Check sheet for the drawn part. Datum: minimum x, y, z corner. Units: mm. A direction names the side the tool comes from. Coordinates: 2 decimals unless noted, no trailing zeros. Loops run counter-clockwise (first coordinate to the right, second up) from the corner with the lowest first, then second, coordinate; pieces in that order, holes last. Notation, with made-up numbers: (75, 50.25) -> (103, 50.25) arc R22 ccw to (103, 72.25) -> close; hole circle Ø1 at (20, 43). An arc over 180 degrees is marked (long way). Use CSV: the item, a comma, the result in double quotes. Start each with the question number.
1. Gauge pin test, flat ends, axial feed: pin 1 (2 mm diameter, centred on x = 54.5, z = 75, fed in from +Y) (3 decimals); pin 2 (18 mm diameter, centred on x = 89, y = 171, fed in from +Z); pin 3 (5 mm diameter, centred on y = 103.5, z = 72, fed in from +X). Record the tip position at first contact, or that the pin passes through.
2. Sectioned sample at B-B, the plane x = 81. Record the cut outline in (y, z).
3. Sectioned sample at D-D, the plane y = 166.5. Record the cut outline in (x, z), and give its area (3 significant figures).
4. Sectioned sample at C-C, the plane z = 75. Record the cut outline in (x, y), and give its area (3 significant figures).
5. Thickness scan on L1, parallel to Y at x = 75, z = 48; L2, parallel to X at y = 330, z = 49; L3, parallel to X at y = 67.5, z = 104. Record the ranges inside material, lowest first.
6. Set-up check for the marked faces 5, 6, 7 and 8: record each of +Z, -Z, +X, -X, +Y, -Y from which the full face is reachable in a straight line by a thin tool's end or side.
7. Release check for a two-part mould opening along Z. For the marked faces 1, 2, 3 and 4 record: pulls with the +Z half, pulls with the -Z half, needs draft (parallel to the pull), parting line crosses it, or undercut.
8. Sectioned sample at A-A, the plane y = 305. Record the cut outline in (x, z), and give its area (3 significant figures).
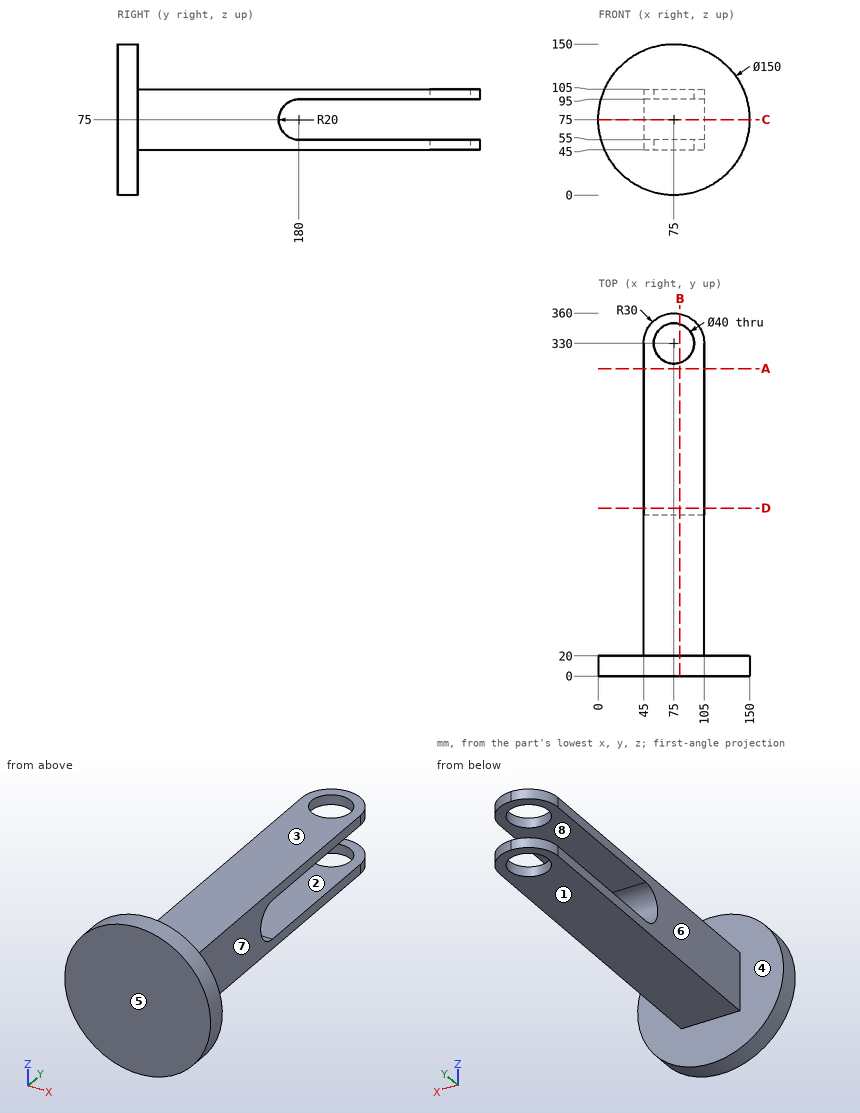
Completed:
1,pin 1,"y = 160.025"
1,pin 2,"z = 105"
1,pin 3,"x = 105"
2,outline,"(0, 0.24) -> (20, 0.24) -> (20, 45) -> (310.92, 45) -> (310.92, 55) -> (180, 55) arc R20 cw to (180, 95) -> (310.92, 95) -> (310.92, 105) -> (20, 105) -> (20, 149.76) -> (0, 149.76) -> close; (349.08, 45) -> (359.39, 45) -> (359.39, 55) -> (349.08, 55) -> close; (349.08, 95) -> (359.39, 95) -> (359.39, 105) -> (349.08, 105) -> close"
3,outline,"(45, 45) -> (105, 45) -> (105, 60.24) -> (45, 60.24) -> close; (45, 89.76) -> (105, 89.76) -> (105, 105) -> (45, 105) -> close"
3,area,"1,830 mm²"
4,outline,"(0, 0) -> (150, 0) -> (150, 20) -> (105, 20) -> (105, 160) -> (45, 160) -> (45, 20) -> (0, 20) -> close"
4,area,"11,400 mm²"
5,L1,"0 to 310, 350 to 360"
5,L2,"45 to 55, 95 to 105"
5,L3,"45 to 105"
6,face 5,"+Z, -Z, +X, -X, -Y"
6,face 6,"+Z, -Z, -X, +Y"
6,face 7,"+Z, -Z, +X, +Y"
6,face 8,"+X, -X, +Y"
7,face 1,"pulls with the -Z half"
7,face 2,"undercut"
7,face 3,"pulls with the +Z half"
7,face 4,"needs draft"
8,outline,"(45, 45) -> (105, 45) -> (105, 55) -> (45, 55) -> close; (45, 95) -> (105, 95) -> (105, 105) -> (45, 105) -> close"
8,area,"1,200 mm²"
